Part print with two shaded views. Sizes in mm from the minimum x, y, z corner. A direction names the side the tool comes from. Round coordinates to 2 decimals unless told otherwise and drop trailing zeros. Order: outer loops, then holes, each group sorted by start corner. A loop starts at its lowest first (then second) coordinate and runs counter-clockwise, first axis right, second up. Notation, with made-up numbers: M 53,-1 L 82,-1 A16 cw 82,4 Z; hole C -5,67 d2. An arc over 180 degrees is marked long. One line per question, with ' | ' between items.
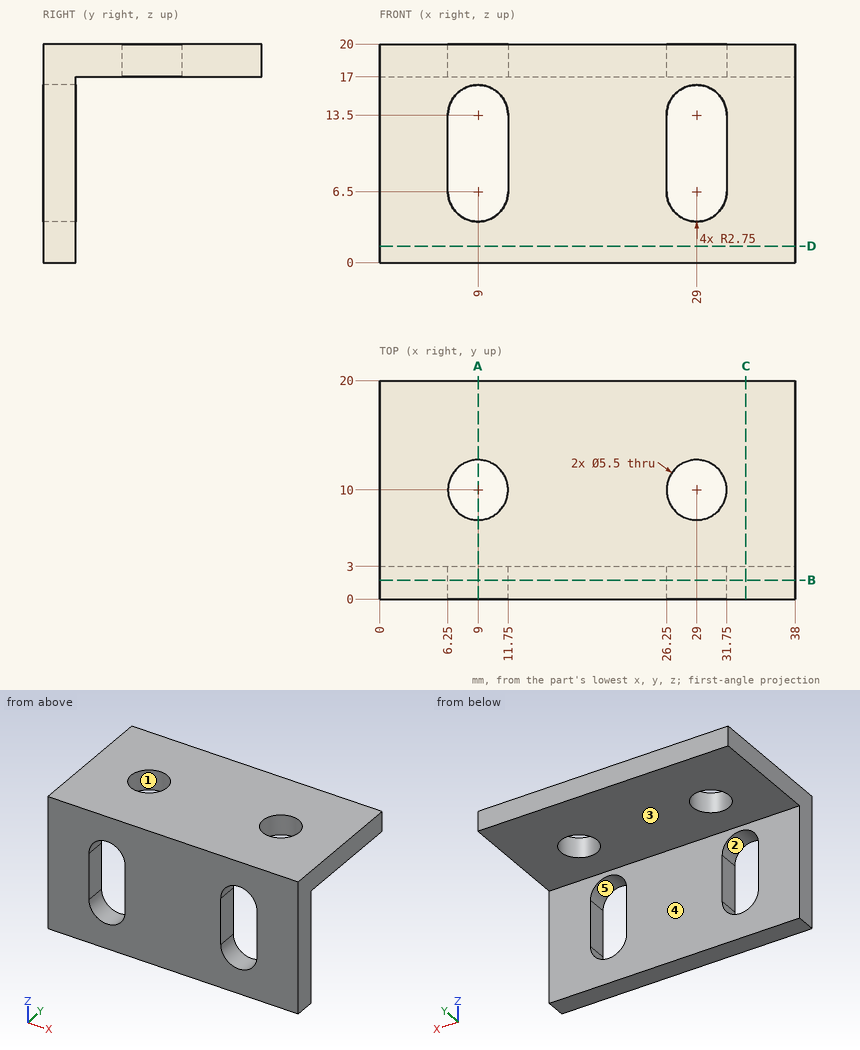
1) Drop flat-ended pins along their axis: pin 1 (6.5 mm diameter, centred on x = 9, y = 10, fed in from +Z); pin 2 (6 mm diameter, centred on y = 7.5, z = 10.5, fed in from -X); pin 3 (8.5 mm diameter, centred on x = 23.5, y = 7.5, fed in from -Z). Give the stop position or say it passes through.
The answers:
pin 1: stops at z = 20 | pin 2: passes through | pin 3: stops at z = 17
2) Saw through at B-B (y = 1.75). List the corners of the cut face in (x, z), plus the area to 3 significant figures.
The answers:
outline: M 0,0 L 38,0 L 38,20 L 0,20 Z; hole M 6.25,6.5 A2.75 ccw 11.75,6.5 L 11.75,13.5 A2.75 ccw 6.25,13.5 Z; hole M 26.25,6.5 A2.75 ccw 31.75,6.5 L 31.75,13.5 A2.75 ccw 26.25,13.5 Z | area: 635 mm²
3) Saw through at A-A (x = 9). List the corners of the cut face in (y, z), plus the area to 3 significant figures.
The answers:
outline: M 0,0 L 3,0 L 3,3.75 L 0,3.75 Z; M 0,16.25 L 3,16.25 L 3,17 L 7.25,17 L 7.25,20 L 0,20 Z; M 12.75,17 L 20,17 L 20,20 L 12.75,20 Z | area: 57.0 mm²
4) Saw through at C-C (x = 33.5). List the corners of the cut face in (y, z), plus the area to 3 significant figures.
The answers:
outline: M 0,0 L 3,0 L 3,17 L 20,17 L 20,20 L 0,20 Z | area: 111 mm²
5) Which spindle directions (+Z, -Z, +X, -X, +Y, -Y) get a long thin tool onto all of the face, cutting with end or side? Do the marked faces 1, 2 and 3. Say none if no direction does.
The answers:
face 1: +Z, -Z | face 2: +Y, -Y | face 3: -Z, +X, -X, +Y
6) Saw through at D-D (z = 1.5). List the corners of the cut face in (x, y), plus the area to 3 significant figures.
The answers:
outline: M 0,0 L 38,0 L 38,3 L 0,3 Z | area: 114 mm²
7) Two-plate mould, pull along X, no slides. Class the marked faces 4 and 5: released by +X, released by -X, zero draft, split by the parting line, or undercut.
The answers:
face 4: zero draft | face 5: undercut
8) Probe line 1 (Y direction, x = 29, z = 18.8); line 2 (X direction, y = 12, z = 18.25); line 3 (Z direction, x = 28.5, y = 19.25). List the from-to ranges inside material, lowest first. Write a range as [from, to].
The answers:
line 1: y = [0, 7.25], [12.75, 20] | line 2: x = [0, 7.11], [10.89, 27.11], [30.89, 38] | line 3: z = [17, 20]
